Geometry check sheet. Reference: the model listing, model coordinates, mm. Give positions to 0.01 mm unless a question says otherwise; leave off trailing zeros. Order: outer loops, then holes, each group sorted by start corner. A loop starts at its lowest first (then second) coordinate and runs counter-clockwise, first axis right, second up. Notation, with made-up numbers: M -19,48.25 L 0,48.25 A18 cw 0,57.25 Z; hole C 59,-21.75 d2. An arc over 180 degrees is marked long. Use CSV: the item, a comma, the result in double quotes. Start each with the question number.
from build123d import *


with BuildPart() as part:
    # Esquisse1 → Révolution2 (revolve)
    with BuildSketch(Plane.XY, mode=Mode.PRIVATE) as r_volution2_sk:
        with BuildLine():
            Line((0, -15), (1.5, -15))
            Line((1.5, -15), (1.5, -7))
            Line((1.5, -7), (3, -7))
            Line((3, -7), (3, -6))
            Line((3, -6), (1, -4.328427125))
            Line((1, -4.328427125), (1, -2.828427125))
            ThreePointArc((1, -2.828427125), (2.956795679, 0.507305936), (0, 3))
            Line((0, 3), (0, -15))
        make_face()
    revolve(r_volution2_sk.sketch.rotate(Axis((0, -15, 0), (0, 1, 0)), 90), axis=Axis((0, -15, 0), (0, 1, 0)))


solid = part.part
(1) Thickness scan on line 1 (Y direction, x = 1, z = -1.25); line 2 (Z direction, x = -2, y = -2); line 3 (Y direction, x = -2, z = -0.5). Record the ranges inside material, lowest first.
(2) Sectioned sample at B-B on y = -9. Record the cut outline in (x, z), then the cut area to 3 significant figures.
(3) Sectioned sample at C-C on y = -0.5. Record the cut outline in (x, z).
(4) Sectioned sample at A-A on z = 0. Record the cut outline in (x, y), then the cut area to 3 significant figures.
(5) Draft check along Y on faces 1 (the face through (1, -4, 0)), 2 (the face through (0, -15, 0)), 3 (the face through (-0.9, -6.49, -2.86)). Enter one of: +Y half, -Y half, draft (parallel to the pull), parting line (faces both ways), or undercut.
(6) Go/stop test with flat-tipped pins: P1, Ø3, axis at x = 2.5, z = 1, coming from the +Y side; P2, Ø1.5, axis at x = 2.5, z = 0, coming from the -Y side; P3, Ø1, axis at x = 1, y = -5.5, coming from the -Z side. Record where each tip stops, or that it passes through.
Responses:
1,line 1,"-7 to -4.83, -2.54 to 2.54"
1,line 2,"-1 to 1"
1,line 3,"-7 to -5.22, -2.18 to 2.18"
2,outline,"C 0,0 d3"
2,area,"7.07 mm2"
3,outline,"C 0,0 d5.92"
4,outline,"M -3,-7 L -1.5,-7 L -1.5,-15 L 1.5,-15 L 1.5,-7 L 3,-7 L 3,-6 L 1,-4.33 L 1,-2.83 A3 ccw long -1,-2.83 L -1,-4.33 L -3,-6 Z"
4,area,"67.7 mm2"
5,face 1,"undercut"
5,face 2,"-Y half"
5,face 3,"draft"
6,P1,"y = 2.75"
6,P2,"y = -7"
6,P3,"z = -2.85"
